The model under review builds one solid part; all positions refer to its coordinate system, in mm. Face numbers are marked on the shaded views. A direction names the side the tool comes from. Coordinates: 2 decimals unless noted, no trailing zeros. Order: outer loops, then holes, each group sorted by start corner. A loop starts at its lowest first (then second) coordinate and runs counter-clockwise, first axis right, second up.
```python
from build123d import *

# Parameters (mm, degrees)
BOSS_EXTRUDE3_DEPTH     = 51
SKETCH2_5_W             = 23
SKETCH2_5_H             = 33
BOSS_EXTRUDE4_DEPTH     = 23.5
SKETCH2_6_W             = 22.5
SKETCH2_6_H             = 33
BOSS_EXTRUDE5_DEPTH     = 41
BOSS_EXTRUDE6_DEPTH     = 31
SKETCH2_8_W             = 4
SKETCH2_8_H             = 16
BOSS_EXTRUDE7_DEPTH     = 75
CUT_EXTRUDE1_DEPTH      = 65
CUT_EXTRUDE1_DEPTH_BACK = 5


with BuildPart() as part:
    # Sketch2 → Boss-Extrude3 (new body)
    with BuildSketch(Plane.XY):
        Polygon((0, 80), (0, 65), (22.5, 65), (45.5, 65), (68, 65), (68, 80), align=None)
    extrude(amount=BOSS_EXTRUDE3_DEPTH)

    # Sketch2_5 → Boss-Extrude4 (add)
    with BuildSketch(Plane.XY):
        with Locations((34, 48.5)):
            Rectangle(SKETCH2_5_W, SKETCH2_5_H)
    extrude(amount=BOSS_EXTRUDE4_DEPTH)

    # Sketch2_6 → Boss-Extrude5 (add)
    with BuildSketch(Plane.XY):
        with Locations((56.75, 48.5)):
            Rectangle(SKETCH2_6_W, SKETCH2_6_H)
        with Locations((11.25, 48.5)):
            Rectangle(SKETCH2_6_W, SKETCH2_6_H)
    extrude(amount=BOSS_EXTRUDE5_DEPTH)

    # Sketch2_7 → Boss-Extrude6 (add)
    with BuildSketch(Plane.XY):
        Polygon((22.5, 32), (0, 32), (0, 16), (4, 16), (4, 0), (64, 0), (64, 16), (68, 16), (68, 32), (45.5, 32), align=None)
    extrude(amount=BOSS_EXTRUDE6_DEPTH)

    # Sketch2_8 → Boss-Extrude7 (add)
    with BuildSketch(Plane.XY):
        with Locations((2, 8)):
            Rectangle(SKETCH2_8_W, SKETCH2_8_H)
        with Locations((66, 8)):
            Rectangle(SKETCH2_8_W, SKETCH2_8_H)
    extrude(amount=BOSS_EXTRUDE7_DEPTH)

    # Sketch9 → Cut-Extrude1 (cut, two sides)
    with BuildSketch(Plane(origin=(4, 0, 0), x_dir=(0, 0, -1), z_dir=(1, 0, 0))) as cut_extrude1_sk:
        with BuildLine():
            Line((-67, 11), (-39, 11))
            ThreePointArc((-39, 11), (-36, 8), (-39, 5))
            Line((-39, 5), (-67, 5))
            ThreePointArc((-67, 5), (-70, 8), (-67, 11))
        make_face()
    extrude(amount=CUT_EXTRUDE1_DEPTH, mode=Mode.SUBTRACT)
    extrude(cut_extrude1_sk.sketch, amount=-CUT_EXTRUDE1_DEPTH_BACK, mode=Mode.SUBTRACT)


solid = part.part
```
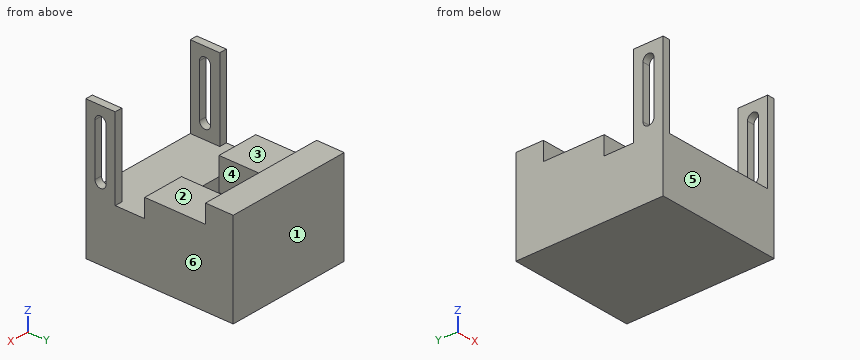
(1) We need section A-A, the plane z = 64.5. Write out the cut boundary in (x, y).
A:
outline: (0, 0) - (4, 0) - (4, 5) - (0, 5) - close; (0, 11) - (4, 11) - (4, 16) - (0, 16) - close; (64, 0) - (68, 0) - (68, 5) - (64, 5) - close; (64, 11) - (68, 11) - (68, 16) - (64, 16) - close
(2) Machinability: for the marked faces 1 and 2, which of the approach directions +Z, -Z, +X, -X, +Y, -Y give a long, thin tool a straight path to every point of the face, cutting with its end or side? Answer none if there is none.
A:
face 1: +Z, -Z, +X, -X, +Y
face 2: +Z, +X, -X
(3) For pin 1 Ø25 at (x, y) = (53.5, 47.5) entering from +Z; pin 2 Ø10 at (x, z) = (19, 40.5) entering from -Y; pin 3 Ø4.5 at (x, y) = (35, 74.5) entering from +Z; pin 4 Ø3 at (y, z) = (39.5, 44) entering from -X, all flat-tipped, find the tip position at first contact; note any pin that passes through.
A:
pin 1: stops at z = 41
pin 2: stops at y = 32
pin 3: stops at z = 51
pin 4: passes through
(4) We need section D-D, the plane y = 42.5. Write out the cut boundary in (x, z).
A:
outline: (0, 0) - (68, 0) - (68, 41) - (45.5, 41) - (45.5, 23.5) - (22.5, 23.5) - (22.5, 41) - (0, 41) - close
(5) Draft analysis for pull direction Y (two halves, no side actions). For the marked faces 3, 4, 5 and 6, state which applies: released by +Y, released by -Y, zero draft, split by the parting line, or undercut.
A:
face 3: undercut
face 4: undercut
face 5: released by -Y
face 6: zero draft
(6) Wall thickness on probe 1 along X at (y, z) = (54, 32); probe 2 along Z at (x, y) = (37.5, 54); probe 3 along Y at (x, z) = (39, 48.5): over which ranges is each line inside the solid? List them lowest first.
A:
probe 1: x = 0 to 22.5, 45.5 to 68
probe 2: z = 0 to 23.5
probe 3: y = 65 to 80
(7) We need section B-B, the plane y = 8. Write out the cut boundary in (x, z).
A:
outline: (0, 0) - (68, 0) - (68, 36) - (64, 36) - (64, 31) - (4, 31) - (4, 36) - (0, 36) - close; (0, 70) - (4, 70) - (4, 75) - (0, 75) - close; (64, 70) - (68, 70) - (68, 75) - (64, 75) - close
(8) We need section C-C, the plane x = 7. Write out the cut boundary in (y, z).
A:
outline: (0, 0) - (80, 0) - (80, 51) - (65, 51) - (65, 41) - (32, 41) - (32, 31) - (0, 31) - close
